```python
from build123d import *

# Parameters (mm, degrees)
SKETCH1_R           = 33
BOSS_EXTRUDE1_DEPTH = 10
SKETCH2_R           = 29.86
BOSS_EXTRUDE2_DEPTH = 30
CUT_EXTRUDE1_DEPTH  = 54
SKETCH4_R           = 4.12
CUT_EXTRUDE2_DEPTH  = 54


with BuildPart() as part:
    # Sketch1 → Boss-Extrude1 (new body)
    with BuildSketch(Plane(origin=(0, 0, 0), x_dir=(1, 0, 0), z_dir=(0, 1, 0))):
        with Locations(Location((0, 0, 0), (0, 0, 270))):
            Circle(SKETCH1_R)
    extrude(amount=BOSS_EXTRUDE1_DEPTH)

    # Sketch2 → Boss-Extrude2 (add)
    with BuildSketch(Plane(origin=(0, 10, 0), x_dir=(1, 0, 0), z_dir=(0, 1, 0))):
        with Locations(Location((0, 0, 0), (0, 0, 270))):
            Circle(SKETCH2_R)
    extrude(amount=BOSS_EXTRUDE2_DEPTH)

    # Sketch3 → Cut-Extrude1 (cut)
    with BuildSketch(Plane(origin=(0, 40, 0), x_dir=(1, 0, 0), z_dir=(0, 1, 0))):
        with BuildLine():
            Line((1.944543648, 20.68287335), (0, 22.627416998))
            Line((0, 22.627416998), (-1.944543648, 20.68287335))
            ThreePointArc((-1.944543648, 20.68287335), (0, 19.877416998), (1.944543648, 20.68287335))
        make_face()
        with BuildLine():
            Line((-1.944543648, 20.68287335), (0, 22.627416998))
            Line((0, 22.627416998), (1.944543648, 20.68287335))
            ThreePointArc((1.944543648, 20.68287335), (2.540668714, 21.575037559), (2.75, 22.627416998))
            ThreePointArc((2.75, 22.627416998), (-1.052379439, 25.168085712), (-1.944543648, 20.68287335))
        make_face()
        with BuildLine():
            ThreePointArc((25.377416998, 0), (23.679796437, 2.540668714), (20.68287335, 1.944543648))
            Line((20.68287335, 1.944543648), (22.627416998, 0))
            Line((22.627416998, 0), (20.68287335, -1.944543648))
            ThreePointArc((20.68287335, -1.944543648), (23.679796437, -2.540668714), (25.377416998, 0))
        make_face()
        with BuildLine():
            Line((22.627416998, 0), (20.68287335, 1.944543648))
            ThreePointArc((20.68287335, 1.944543648), (19.877416998, 0), (20.68287335, -1.944543648))
            Line((20.68287335, -1.944543648), (22.627416998, 0))
        make_face()
        with BuildLine():
            ThreePointArc((1.944543648, -20.68287335), (0, -19.877416998), (-1.944543648, -20.68287335))
            Line((-1.944543648, -20.68287335), (0, -22.627416998))
            Line((0, -22.627416998), (1.944543648, -20.68287335))
        make_face()
        with BuildLine():
            Line((0, -22.627416998), (-1.944543648, -20.68287335))
            ThreePointArc((-1.944543648, -20.68287335), (-1.052379439, -25.168085712), (2.75, -22.627416998))
            ThreePointArc((2.75, -22.627416998), (2.540668714, -21.575037559), (1.944543648, -20.68287335))
            Line((1.944543648, -20.68287335), (0, -22.627416998))
        make_face()
        with BuildLine():
            ThreePointArc((-19.877416998, 0), (-20.086748284, 1.052379439), (-20.68287335, 1.944543648))
            Line((-20.68287335, 1.944543648), (-22.627416998, 0))
            Line((-22.627416998, 0), (-20.68287335, -1.944543648))
            ThreePointArc((-20.68287335, -1.944543648), (-20.086748284, -1.052379439), (-19.877416998, 0))
        make_face()
        with BuildLine():
            Line((-22.627416998, 0), (-20.68287335, 1.944543648))
            ThreePointArc((-20.68287335, 1.944543648), (-25.377416998, 0), (-20.68287335, -1.944543648))
            Line((-20.68287335, -1.944543648), (-22.627416998, 0))
        make_face()
    extrude(amount=-CUT_EXTRUDE1_DEPTH, mode=Mode.SUBTRACT)

    # Sketch4 → Cut-Extrude2 (cut)
    with BuildSketch(Plane(origin=(0, 40, 0), x_dir=(1, 0, 0), z_dir=(0, 1, 0))):
        Circle(SKETCH4_R)
        with BuildLine():
            Line((0, 5.44), (0, 4.12))
            ThreePointArc((0, 4.12), (0.789638797, 4.043620973), (1.55, 3.817315811))
            Line((1.55, 3.817315811), (1.55, 5.44))
            Line((1.55, 5.44), (0, 5.44))
        make_face()
        with BuildLine():
            ThreePointArc((-1.55, 3.817315811), (-0.789638797, 4.043620973), (0, 4.12))
            Line((0, 4.12), (0, 5.44))
            Line((0, 5.44), (-1.55, 5.44))
            Line((-1.55, 5.44), (-1.55, 3.817315811))
        make_face()
    extrude(amount=-CUT_EXTRUDE2_DEPTH, mode=Mode.SUBTRACT)


solid = part.part
```
Work out the finished part from the listing and answer in its coordinate system (mm). A direction names the side the tool comes from. Coordinates: 2 decimals unless noted, no trailing zeros. Loops run counter-clockwise (first coordinate to the right, second up) from the corner with the lowest first, then second, coordinate; pieces in that order, holes last.
1) Section A-A (x = 0) is taken. Give the vertices of the cut face in (y, z), plus the area to 3 significant figures.
Results:
outline: (0, -33) - (10, -33) - (10, -29.86) - (40, -29.86) - (40, -25.38) - (0, -25.38) - close; (0, -19.88) - (40, -19.88) - (40, -5.44) - (0, -5.44) - close; (0, 4.12) - (40, 4.12) - (40, 19.88) - (0, 19.88) - close; (0, 25.38) - (40, 25.38) - (40, 29.86) - (10, 29.86) - (10, 33) - (0, 33) - close
area: 1,630 mm2
2) Section D-D (z = 17) is taken. Give the vertices of the cut face in (x, y), plus the area to 3 significant figures.
Results:
outline: (-28.28, 0) - (28.28, 0) - (28.28, 10) - (24.55, 10) - (24.55, 40) - (-24.55, 40) - (-24.55, 10) - (-28.28, 10) - close
area: 2,040 mm2
3) Flat-ended cylindrical pins translate along their axes: pin 1 (6.5 mm diameter, centred on x = 0, z = 0, fed in from -Y); pin 2 (6 mm diameter, centred on x = -17.5, y = 31.5, fed in from +Z); pin 3 (3 mm diameter, centred on x = 8.5, y = 5.5, fed in from -Z); pin 4 (3.5 mm diameter, centred on x = 0, y = 28, fed in from +Z). Find the tip coordinate at first contact, or state that the pin passes through.
Results:
pin 1: passes through
pin 2: stops at z = 26.1
pin 3: stops at z = -32.25
pin 4: stops at z = 29.86
4) Section B-B (y = 21.5) is taken. Give the vertices of the cut face in (x, z), plus the area to 3 significant figures.
Results:
outline: circle Ø59.72 at (0, 0); hole circle Ø5.5 at (-22.63, 0); hole circle Ø5.5 at (0, -22.63); hole circle Ø5.5 at (0, 22.63); hole (-1.55, -5.44) - (1.55, -5.44) - (1.55, -3.82) arc R4.12 ccw (long way) to (-1.55, -3.82) - close; hole circle Ø5.5 at (22.63, 0)
area: 2,650 mm2
5) Section C-C (y = 8) is taken. Give the vertices of the cut face in (x, z).
Results:
outline: circle Ø66 at (0, 0); hole circle Ø5.5 at (-22.63, 0); hole circle Ø5.5 at (0, -22.63); hole circle Ø5.5 at (0, 22.63); hole (-1.55, -5.44) - (1.55, -5.44) - (1.55, -3.82) arc R4.12 ccw (long way) to (-1.55, -3.82) - close; hole circle Ø5.5 at (22.63, 0)
6) Consider probe 1 along X at (y, z) = (9.5, 0); probe 2 along X at (y, z) = (31, 0); probe 3 along Z at (x, y) = (2, 6). Determine where each line is inside the solid, lowest interval first.
Results:
probe 1: x = -33 to -25.38, -19.88 to -4.12, 4.12 to 19.88, 25.38 to 33
probe 2: x = -29.86 to -25.38, -19.88 to -4.12, 4.12 to 19.88, 25.38 to 29.86
probe 3: z = -32.94 to -24.51, -20.74 to -3.6, 3.6 to 20.74, 24.51 to 32.94
7) For a pull along Z with two mould halves and no side action, classify faces 4 (the cylindrical face through (-32.215, 4.93, -7.154)), 5 (the cylindrical face through (-0.159, 20.28, 4.117)), 6 (the flat face through (0, 20, -5.44)), 7 (the flat face through (-17, 10, -25)) as +Z half, -Z half, draft (parallel to the pull), parting line (faces both ways), or undercut.
Results:
face 4: parting line
face 5: undercut
face 6: undercut
face 7: draft
8) For faces 1 (the cylindrical face through (-18.169, 24.79, -23.696)), 2 (the flat face through (-7, 0, 0)), 3 (the flat face through (-1.55, 20, -5)), determine the directions among +Z, -Z, +X, -X, +Y, -Y from which every point of the face is accessible in a straight line to the end or side of a thin tool.
Results:
face 1: +Y
face 2: +Z, -Z, +X, -X, -Y
face 3: +Y, -Y
